Can you work these out from the model? Positions are in its coordinate system, mm. Face numbers are marked on the shaded views. Round coordinates to 2 decimals unless told otherwise and drop trailing zeros. Loops run counter-clockwise (first coordinate to the right, second up) from the corner with the lowest first, then second, coordinate; pieces in that order, holes last. Notation, with made-up numbers: (22.5, -36) -> (36.5, -36) arc R17 ccw to (36.5, -26) -> close; hole circle Ø3 at (24.25, -2.5). An arc over 180 degrees is marked (long way). Use a Markdown table: item, result.
from build123d import *

# Parameters (mm, degrees)
SCHIZZO1_R                   = 3
SCHIZZO1_R_2                 = 1.5
ESTRUSIONE_ESTRUSIONE1_DEPTH = 10
SMUSSO1_SIZE                 = 0.5
CHAMFER1_SIZE                = 0.5


with BuildPart() as part:
    # Schizzo1 → Estrusione-Estrusione1 (new body)
    with BuildSketch(Plane.XY):
        Circle(SCHIZZO1_R)
        Circle(SCHIZZO1_R_2, mode=Mode.SUBTRACT)
    extrude(amount=ESTRUSIONE_ESTRUSIONE1_DEPTH)

    # Smusso1
    smusso1_edges = [part.edges().sort_by_distance(p)[0] for p in [
        (-1.5, 0, 10),
    ]]
    chamfer(smusso1_edges, length=SMUSSO1_SIZE)

    # Chamfer1
    chamfer1_edges = [part.edges().sort_by_distance(p)[0] for p in [
        (-1.5, 0, 0),
    ]]
    chamfer(chamfer1_edges, length=CHAMFER1_SIZE)


solid = part.part
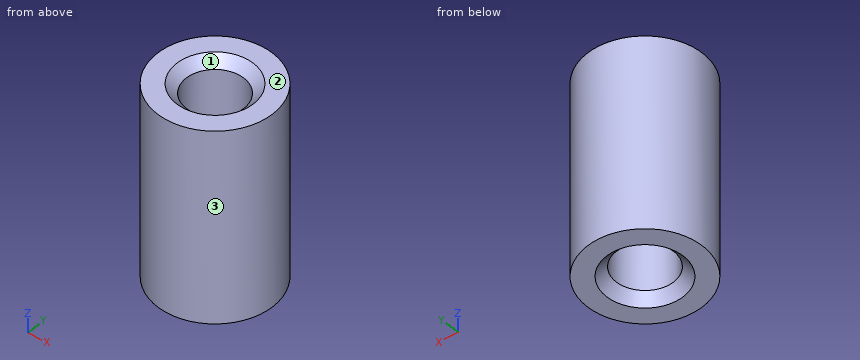
1. I want a section at A-A (y = 0). Please give me the cut outline in (x, z), plus the area to 3 significant figures.
Answer sheet:
| item | result |
|---|---|
| outline | (-3, 0) -> (-2, 0) -> (-1.5, 0.5) -> (-1.5, 9.5) -> (-2, 10) -> (-3, 10) -> close; (1.5, 0.5) -> (2, 0) -> (3, 0) -> (3, 10) -> (2, 10) -> (1.5, 9.5) -> close |
| area | 29.5 mm² |
2. I want a section at C-C (z = 5.5). Please give me the cut outline in (x, y), plus the area to 3 significant figures.
Answer sheet:
| item | result |
|---|---|
| outline | circle Ø6 at (0, 0); hole circle Ø3 at (0, 0) |
| area | 21.2 mm² |
3. If we mould it in two halves opening along Y, with no side actions, what happens to the marked faces 1, 2 and 3? For each: +Y half, -Y half, draft (parallel to the pull), parting line (faces both ways), or undercut.
Answer sheet:
| item | result |
|---|---|
| face 1 | undercut |
| face 2 | draft |
| face 3 | parting line |
4. Will these pins go through, and if not, where does the flat tip stop? pin 1 Ø1.5 at (y, z) = (-1, 8.5) entering from +X; pin 2 Ø2 at (x, y) = (-1.5, -1) entering from +Z.
Answer sheet:
| item | result |
|---|---|
| pin 1 | stops at x = 2.99 |
| pin 2 | stops at z = 10 |
5. I want a section at D-D (y = 2.25). Please give me the cut outline in (x, z).
Answer sheet:
| item | result |
|---|---|
| outline | (-1.98, 0) -> (1.98, 0) -> (1.98, 10) -> (-1.98, 10) -> close |
6. I need wall thicknesses on line 1 (Y direction, x = 0, z = 3.25); line 2 (Y direction, x = 0.6, z = 7); line 3 (X direction, y = 2.6, z = 4). Which ranges of each line are inside material? Lowest first, please.
Answer sheet:
| item | result |
|---|---|
| line 1 | y = -3 to -1.5, 1.5 to 3 |
| line 2 | y = -2.94 to -1.37, 1.37 to 2.94 |
| line 3 | x = -1.5 to 1.5 |
